from build123d import *

# Parameters (mm, degrees)
PAD_DEPTH         = 5
POCKET_DEPTH      = 4
POCKET_FACE1_W    = 7
POCKET_FACE1_H    = 5
PAD001_DEPTH      = 3
PAD001_FACE6_W    = 7
PAD001_FACE6_H    = 5
PAD002_DEPTH      = 3
PAD002_FACE6_W    = 7
PAD002_FACE6_H    = 5
PAD003_DEPTH      = 3
PAD003_FACE1_W    = 7
PAD003_FACE1_H    = 5
PAD004_DEPTH      = 3
PAD004_FACE1_W    = 7
PAD004_FACE1_H    = 5
PAD005_DEPTH      = 3
PAD005_FACE1_W    = 7
PAD005_FACE1_H    = 5
PAD006_DEPTH      = 3
FILLET_R          = 1
FILLET001_R       = 0.7
SKETCH002_R       = 1.5
POCKET001_DEPTH   = 5
POCKET001_FACE5_R = 1.5
PAD007_DEPTH      = 0.5


with BuildPart() as part:
    # Sketch → Pad (new body)
    with BuildSketch(Plane.XY):
        Polygon((7, 0), (3.5, 6.0621778265), (-3.5, 6.0621778265), (-7, 0), (-3.5, -6.0621778265), (3.5, -6.0621778265), align=None)
    extrude(amount=PAD_DEPTH)

    # Sketch001 (on Face7 of Pad) → Pocket (cut)
    with BuildSketch(Plane(origin=(0, 0, 0), x_dir=(1, 0, 0), z_dir=(0, 0, -1))):
        Polygon((3.35, 0), (1.675, 2.9011851027), (-1.675, 2.9011851027), (-3.35, 0), (-1.675, -2.9011851027), (1.675, -2.9011851027), align=None)
    extrude(amount=-POCKET_DEPTH, mode=Mode.SUBTRACT)

    # Pocket Face1 → Pad001 (add)
    with BuildSketch(Plane(origin=(5.25, 3.0310889132, 2.5), x_dir=(0.5, -0.8660254038, 0), z_dir=(0.8660254038, 0.5, 0))):
        Rectangle(POCKET_FACE1_W, POCKET_FACE1_H)
    extrude(amount=PAD001_DEPTH)

    # Pad001 Face6 → Pad002 (add)
    with BuildSketch(Plane(origin=(-5.25, -3.0310889132, 2.5), x_dir=(-0.5, 0.8660254038, 0), z_dir=(-0.8660254038, -0.5, 0))):
        Rectangle(PAD001_FACE6_W, PAD001_FACE6_H)
    extrude(amount=PAD002_DEPTH)

    # Pad002 Face6 → Pad003 (add)
    with BuildSketch(Plane(origin=(-5.25, 3.0310889132, 2.5), x_dir=(0.5, 0.8660254038, 0), z_dir=(-0.8660254038, 0.5, 0))):
        Rectangle(PAD002_FACE6_W, PAD002_FACE6_H)
    extrude(amount=PAD003_DEPTH)

    # Pad003 Face1 → Pad004 (add)
    with BuildSketch(Plane(origin=(0, 6.0621778265, 2.5), x_dir=(1, 0, 0), z_dir=(0, 1, 0))):
        Rectangle(PAD003_FACE1_W, PAD003_FACE1_H)
    extrude(amount=PAD004_DEPTH)

    # Pad004 Face1 → Pad005 (add)
    with BuildSketch(Plane(origin=(5.25, -3.0310889132, 2.5), x_dir=(-0.5, -0.8660254038, 0), z_dir=(0.8660254038, -0.5, 0))):
        Rectangle(PAD004_FACE1_W, PAD004_FACE1_H)
    extrude(amount=PAD005_DEPTH)

    # Pad005 Face1 → Pad006 (add)
    with BuildSketch(Plane(origin=(0, -6.0621778265, 2.5), x_dir=(-1, 0, 0), z_dir=(0, -1, 0))):
        Rectangle(PAD005_FACE1_W, PAD005_FACE1_H)
    extrude(amount=PAD006_DEPTH)

    # Fillet
    fillet_edges = [part.edges().sort_by_distance(p)[0] for p in [
        (3.5, -6.062178, 2.5),
        (-3.5, -6.062178, 2.5),
        (-7, 0, 2.5),
        (-3.5, 6.062178, 2.5),
        (3.5, 6.062178, 2.5),
        (7, 0, 2.5),
    ]]
    fillet(fillet_edges, radius=FILLET_R)

    # Fillet001
    fillet001_edges = [part.edges().sort_by_distance(p)[0] for p in [
        (-6.098076, -7.562178, 2.5),
        (-9.598076, -1.5, 2.5),
        (-9.598076, 1.5, 2.5),
        (-6.098076, 7.562178, 2.5),
        (-3.5, 9.062178, 2.5),
        (3.5, 9.062178, 2.5),
        (6.098076, 7.562178, 2.5),
        (9.598076, 1.5, 2.5),
        (9.598076, -1.5, 2.5),
        (6.098076, -7.562178, 2.5),
        (3.5, -9.062178, 2.5),
        (-3.5, -9.062178, 2.5),
    ]]
    fillet(fillet001_edges, radius=FILLET001_R)

    # Sketch002 (on Face45 of Fillet001) → Pocket001 (cut)
    with BuildSketch(Plane(origin=(0, 0, 4), x_dir=(1, 0, 0), z_dir=(0, 0, -1))):
        Circle(SKETCH002_R)
    extrude(amount=-POCKET001_DEPTH, mode=Mode.SUBTRACT)

    # Pocket001 Face5 → Pad007 (add)
    with BuildSketch(Plane(origin=(0, 0, 5), x_dir=(0, 1, 0), z_dir=(0, 0, 1))):
        with BuildLine():
            Line((6.9282032303, 5), (7.2121778265, 5.4918584287))
            ThreePointArc((7.2121778265, 5.4918584287), (7.2821081222, 6.0230317603), (6.9559600438, 6.4480762114))
            Line((6.9559600438, 6.4480762114), (2.1062177826, 9.2480762114))
            ThreePointArc((2.1062177826, 9.2480762114), (1.5750444511, 9.3180065071), (1.15, 8.9918584287))
            Line((1.15, 8.9918584287), (0.8660254038, 8.5))
            ThreePointArc((0.8660254038, 8.5), (0, 8), (-0.8660254038, 8.5))
            Line((-0.8660254038, 8.5), (-1.15, 8.9918584287))
            ThreePointArc((-1.15, 8.9918584287), (-1.5750444511, 9.3180065071), (-2.1062177826, 9.2480762114))
            Line((-2.1062177826, 9.2480762114), (-6.9559600438, 6.4480762114))
            ThreePointArc((-6.9559600438, 6.4480762114), (-7.2821081222, 6.0230317603), (-7.2121778265, 5.4918584287))
            Line((-7.2121778265, 5.4918584287), (-6.9282032303, 5))
            ThreePointArc((-6.9282032303, 5), (-6.9282032303, 4), (-7.7942286341, 3.5))
            Line((-7.7942286341, 3.5), (-8.3621778265, 3.5))
            ThreePointArc((-8.3621778265, 3.5), (-8.8571525733, 3.2949747468), (-9.0621778265, 2.8))
            Line((-9.0621778265, 2.8), (-9.0621778265, -2.8))
            ThreePointArc((-9.0621778265, -2.8), (-8.8571525733, -3.2949747468), (-8.3621778265, -3.5))
            Line((-8.3621778265, -3.5), (-7.7942286341, -3.5))
            ThreePointArc((-7.7942286341, -3.5), (-6.9282032303, -4), (-6.9282032303, -5))
            Line((-6.9282032303, -5), (-7.2121778265, -5.4918584287))
            ThreePointArc((-7.2121778265, -5.4918584287), (-7.2821081222, -6.0230317603), (-6.9559600438, -6.4480762114))
            Line((-6.9559600438, -6.4480762114), (-2.1062177826, -9.2480762114))
            ThreePointArc((-2.1062177826, -9.2480762114), (-1.5750444511, -9.3180065071), (-1.15, -8.9918584287))
            Line((-1.15, -8.9918584287), (-0.8660254038, -8.5))
            ThreePointArc((-0.8660254038, -8.5), (0, -8), (0.8660254038, -8.5))
            Line((0.8660254038, -8.5), (1.15, -8.9918584287))
            ThreePointArc((1.15, -8.9918584287), (1.5750444511, -9.3180065071), (2.1062177826, -9.2480762114))
            Line((2.1062177826, -9.2480762114), (6.9559600438, -6.4480762114))
            ThreePointArc((6.9559600438, -6.4480762114), (7.2821081222, -6.0230317603), (7.2121778265, -5.4918584287))
            Line((7.2121778265, -5.4918584287), (6.9282032303, -5))
            ThreePointArc((6.9282032303, -5), (6.9282032303, -4), (7.7942286341, -3.5))
            Line((7.7942286341, -3.5), (8.3621778265, -3.5))
            ThreePointArc((8.3621778265, -3.5), (8.8571525733, -3.2949747468), (9.0621778265, -2.8))
            Line((9.0621778265, -2.8), (9.0621778265, 2.8))
            ThreePointArc((9.0621778265, 2.8), (8.8571525733, 3.2949747468), (8.3621778265, 3.5))
            Line((8.3621778265, 3.5), (7.7942286341, 3.5))
            ThreePointArc((7.7942286341, 3.5), (6.9282032303, 4), (6.9282032303, 5))
        make_face()
        Circle(POCKET001_FACE5_R, mode=Mode.SUBTRACT)
    extrude(amount=PAD007_DEPTH)


solid = part.part
Can you work these out from the model? Positions are in its coordinate system, mm. A direction names the side the tool comes from. Give positions to 0.01 mm unless a question says otherwise; leave off trailing zeros. Loops run counter-clockwise (first coordinate to the right, second up) from the corner with the lowest first, then second, coordinate; pieces in that order, holes last. Notation, with made-up numbers: (-1.5, -13.5) -> (37.5, -13.5) arc R20 ccw to (37.5, 18.5) -> close; hole circle Ø6 at (83, -1). An arc over 180 degrees is marked (long way). Write item = value, one per line.
1) Suppose I cut it at D-D on x = 3.75. Write out the boundary of the cut face in (y, z), then the cut area to 3 significant figures.
Check result:
outline = (-7.13, 0) -> (7.13, 0) -> (7.13, 5.5) -> (-7.13, 5.5) -> close
area = 78.5 mm2
2) Will these pins go through, and if not, where does the flat tip stop? pin 1 (1.5 mm diameter, centred on y = -6, z = 1, fed in from -X); pin 2 (5 mm diameter, centred on x = 0, y = 0, fed in from -Z); pin 3 (0.6 mm diameter, centred on y = 8, z = 2.5, fed in from -X).
Check result:
pin_1 = -7.43
pin_2 = 4
pin_3 = -3.5
3) Thinking about a two-plate mould opening in X: for faces 3 (the flat face through (0, 2.901, 2)), 4 (the flat face through (0, 9.062, 3)), which applies, released by +X, released by -X, zero draft, split by the parting line, or undercut?
Check result:
face_3 = undercut
face_4 = zero draft
4) Suppose I cut it at B-B on y = -0.25. Write out the boundary of the cut face in (x, z), then the cut area to 3 significant figures.
Check result:
outline = (-8.03, 0) -> (-3.21, 0) -> (-3.21, 4) -> (-1.48, 4) -> (-1.48, 5.5) -> (-8.03, 5.5) -> close; (1.48, 4) -> (3.21, 4) -> (3.21, 0) -> (8.03, 0) -> (8.03, 5.5) -> (1.48, 5.5) -> close
area = 58.3 mm2
5) Suppose I cut it at A-A on x = 0. Write out the boundary of the cut face in (y, z).
Check result:
outline = (-9.06, 0) -> (-2.9, 0) -> (-2.9, 4) -> (-1.5, 4) -> (-1.5, 5.5) -> (-9.06, 5.5) -> close; (1.5, 4) -> (2.9, 4) -> (2.9, 0) -> (9.06, 0) -> (9.06, 5.5) -> (1.5, 5.5) -> close
6) For faces 1 (the flat face through (0, -4, 0)), 2 (the flat face through (0, -2.901, 2)), which set-ups out of +Z, -Z, +X, -X, +Y, -Y let a thin tool reach every point of the face, with its end or its side?
Check result:
face_1 = -Z, +X, -X, +Y, -Y
face_2 = -Z
7) I need wall thicknesses on L1, parallel to Y at x = 0, z = 5.1; L2, parallel to Y at x = -1.25, z = 3.95; L3, parallel to Y at x = -5.75, z = 0.9. Which ranges of each line are inside material? Lowest first, please. Write a range as from..to.
Check result:
L1 = -9.06..-1.5, 1.5..9.06
L2 = -9.06..-2.9, 2.9..9.06
L3 = -7.3..7.3
8) Suppose I cut it at C-C on y = 5.75. Write out the boundary of the cut face in (x, z).
Check result:
outline = (-7.14, 0) -> (7.14, 0) -> (7.14, 5.5) -> (-7.14, 5.5) -> close
